from build123d import *

# Parameters (mm, degrees)
SKETCH_1_W          = 24
SKETCH_1_H          = 24
EXTRUDE_2_DEPTH     = 20
SKETCH_3_W          = 21
SKETCH_3_H          = 21
CUT_EXTRUDE_1_DEPTH = 20
SKETCH_4_W          = 24
SKETCH_4_H          = 3
EXTRUDE_8_DEPTH     = 2
SKETCH_8_W          = 3
SKETCH_8_H          = 21
EXTRUDE_9_DEPTH     = 2
SKETCH_9_W          = 21
SKETCH_9_H          = 3
EXTRUDE_10_DEPTH    = 2
SKETCH_10_W         = 3
SKETCH_10_H         = 18
EXTRUDE_11_DEPTH    = 2
SKETCH_11_W         = 24
SKETCH_11_H         = 23
EXTRUDE_12_DEPTH    = 4
CUT_EXTRUDE_2_DEPTH = 4


with BuildPart() as part:
    # 草图1 → 凸台-拉伸2 (new body)
    with BuildSketch(Plane.XY):
        Rectangle(SKETCH_1_W, SKETCH_1_H)
    extrude(amount=EXTRUDE_2_DEPTH)

    # 草图3 → 切除-拉伸1 (cut)
    with BuildSketch(Plane.XY.offset(20)):
        Rectangle(SKETCH_3_W, SKETCH_3_H)
    extrude(amount=-CUT_EXTRUDE_1_DEPTH, mode=Mode.SUBTRACT)

    # 草图4 → 凸台-拉伸8 (add)
    with BuildSketch(Plane.XY.offset(20)):
        with Locations((0, 10.5)):
            Rectangle(SKETCH_4_W, SKETCH_4_H)
    extrude(amount=EXTRUDE_8_DEPTH)

    # 草图8 → 凸台-拉伸9 (add)
    with BuildSketch(Plane.XY.offset(20)):
        with Locations((-10.5, -1.5)):
            Rectangle(SKETCH_8_W, SKETCH_8_H)
    extrude(amount=EXTRUDE_9_DEPTH)

    # 草图9 → 凸台-拉伸10 (add)
    with BuildSketch(Plane.XY.offset(20)):
        with Locations((1.5, -10.5)):
            Rectangle(SKETCH_9_W, SKETCH_9_H)
    extrude(amount=EXTRUDE_10_DEPTH)

    # 草图10 → 凸台-拉伸11 (add)
    with BuildSketch(Plane.XY.offset(20)):
        with Locations((10.5, 0)):
            Rectangle(SKETCH_10_W, SKETCH_10_H)
    extrude(amount=EXTRUDE_11_DEPTH)

    # 草图11 → 凸台-拉伸12 (add)
    with BuildSketch(Plane.XY.offset(22)):
        with Locations((0, -11.5)):
            Rectangle(SKETCH_11_W, SKETCH_11_H)
    extrude(amount=EXTRUDE_12_DEPTH)

    # 草图12 → 切除-拉伸2 (cut)
    with BuildSketch(Plane.XY.offset(26)):
        with BuildLine():
            Line((-3.5, -14), (-3.5, -20))
            ThreePointArc((-3.5, -20), (-5, -21.5), (-6.5, -20))
            Line((-6.5, -20), (-6.5, -14))
            ThreePointArc((-6.5, -14), (-5, -12.5), (-3.5, -14))
        make_face()
        with BuildLine():
            Line((3.5, -14), (3.5, -20))
            ThreePointArc((3.5, -20), (5, -21.5), (6.5, -20))
            Line((6.5, -20), (6.5, -14))
            ThreePointArc((6.5, -14), (5, -12.5), (3.5, -14))
        make_face()
    extrude(amount=-CUT_EXTRUDE_2_DEPTH, mode=Mode.SUBTRACT)


solid = part.part
For this review, take the finished solid that the model builds, in its own axes (mm). A direction names the side the tool comes from. Give positions to 0.01 mm unless a question says otherwise; leave off trailing zeros. Loops run counter-clockwise (first coordinate to the right, second up) from the corner with the lowest first, then second, coordinate; pieces in that order, holes last. Notation, with made-up numbers: M 17,-10.75 L 66,-10.75 A19 ccw 66,5.25 Z; hole C 54,39.25 d8. An arc over 180 degrees is marked long. Answer as a JSON object with one key per item and string values. Group by question number.
Q1. Tool access review of faces 4 (the flat face through (0, 10.5, 10)), 5 (the cylindrical face through (-5, -12.5, 24)), 6 (the flat face through (-11, 0, 0)), 7 (the flat face through (0, 0, 24)), 8 (the flat face through (12, -2, 13)): name each direction out of +Z, -Z, +X, -X, +Y, -Y from which nothing blocks a thin tool from reaching the whole face with its end or side.
Q2. Mouldability with a two-part tool opening along Y and no side actions: class faces 1 (the flat face through (0, -17, 22)), 2 (the flat face through (0, -12, 11)), 3 (the flat face through (-10.5, 0, 10)) as +Y half, -Y half, draft (parallel to the pull), parting line (faces both ways), or undercut.
Q3. Add section C-C on x = -0.75. Give the boundary of the cut face in (y, z), and give its area (3 significant figures).
Q4. Insertion check: P1, Ø12, axis at x = -3.5, y = 7, coming from the -Z side; P2, Ø2.5, axis at x = -1.5, y = -5.5, coming from the -Z side; P3, Ø8, axis at x = 6, z = 15.5, coming from the -Y side; P4, Ø1.5, axis at x = 7.5, y = -9, coming from the -Z side. Each pin has a flat end and moves straight along its axis. Give the tip position at first contact, or say it passes through.
Q5. For probe 1 along X at (y, z) = (7.5, 21); probe 2 along Y at (x, z) = (3.75, 17.25), list the stretches that pass through material, from the lowest coordinate up. Write a range as [from, to].
Q6. Add section D-D on z = 18. Give the boundary of the cut face in (x, y), and give its area (3 significant figures).
Q7. Add section A-A on y = 7. Give the boundary of the cut face in (x, z).
Q8. Add section B-B on x = 5. Give the boundary of the cut face in (y, z).
Checked values:
{
 "1": {"face 4": "-Z", "face 5": "+Z, -Z", "face 6": "-Z, +X, -X, +Y, -Y", "face 7": "+Z, +X, -X, +Y", "face 8": "+Z, -Z, +X, +Y, -Y"},
 "2": {"face 1": "draft", "face 2": "-Y half", "face 3": "undercut"},
 "3": {"outline": "M -23,22 L -12,22 L -12,0 L -10.5,0 L -10.5,20 L -9,20 L -9,22 L 0,22 L 0,26 L -23,26 Z; M 9,20 L 10.5,20 L 10.5,0 L 12,0 L 12,22 L 9,22 Z", "area": "164 mm²"},
 "4": {"P1": "z = 0", "P2": "z = 22", "P3": "y = -12", "P4": "z = 20"},
 "5": {"probe 1": "[-12, -9], [9, 12]", "probe 2": "[-12, -10.5], [10.5, 12]"},
 "6": {"outline": "M -12,-12 L 12,-12 L 12,12 L -12,12 Z; hole M -10.5,-10.5 L 10.5,-10.5 L 10.5,10.5 L -10.5,10.5 Z", "area": "135 mm²"},
 "7": {"outline": "M -12,0 L -10.5,0 L -10.5,20 L -9,20 L -9,22 L -12,22 Z; M 9,20 L 10.5,20 L 10.5,0 L 12,0 L 12,22 L 9,22 Z"},
 "8": {"outline": "M -23,22 L -21.5,22 L -21.5,26 L -23,26 Z; M -12.5,22 L -12,22 L -12,0 L -10.5,0 L -10.5,20 L -9,20 L -9,22 L 0,22 L 0,26 L -12.5,26 Z; M 9,20 L 10.5,20 L 10.5,0 L 12,0 L 12,22 L 9,22 Z"}
}
